from build123d import *

# Parameters (mm, degrees)
SKETCH1_R           = 1.75
BOSS_EXTRUDE1_DEPTH = 3
SKETCH2_W           = 5
SKETCH2_H           = 8
BOSS_EXTRUDE2_DEPTH = 12
BOSS_EXTRUDE3_DEPTH = 8
FILLET2_R           = 8


with BuildPart() as part:
    # Sketch1 → Boss-Extrude1 (new body)
    with BuildSketch(Plane(origin=(0, 0, 0), x_dir=(1, 0, 0), z_dir=(0, 1, 0))):
        with BuildLine():
            Line((-11.25, -4), (11.25, -4))
            ThreePointArc((11.25, -4), (15.25, 0), (11.25, 4))
            Line((11.25, 4), (-11.25, 4))
            ThreePointArc((-11.25, 4), (-15.25, 0), (-11.25, -4))
        make_face()
        with Locations((-11.25, 0)):
            Circle(SKETCH1_R, mode=Mode.SUBTRACT)
        with Locations((11.25, 0)):
            Circle(SKETCH1_R, mode=Mode.SUBTRACT)
    extrude(amount=BOSS_EXTRUDE1_DEPTH)

    # Sketch2 → Boss-Extrude2 (add)
    with BuildSketch(Plane(origin=(0, 3, 0), x_dir=(1, 0, 0), z_dir=(0, 1, 0))):
        with Locations((3.75, 0)):
            Rectangle(SKETCH2_W, SKETCH2_H)
    extrude(amount=BOSS_EXTRUDE2_DEPTH)

    # Sketch3 → Boss-Extrude3 (add)
    with BuildSketch(Plane.XY.offset(4)):
        Polygon((1.25, 15), (-6.25, 3), (1.25, 3), align=None)
    extrude(amount=-BOSS_EXTRUDE3_DEPTH)

    # Fillet2
    fillet2_edges = [part.edges().sort_by_distance(p)[0] for p in [
        (1.25, 15, 0),
    ]]
    fillet(fillet2_edges, radius=FILLET2_R)


solid = part.part
For this review, take the finished solid that the model builds, in its own axes (mm). A direction names the side the tool comes from. Give positions to 0.01 mm unless a question says otherwise; leave off trailing zeros. Loops run counter-clockwise (first coordinate to the right, second up) from the corner with the lowest first, then second, coordinate; pieces in that order, holes last. Notation, with made-up numbers: M 52.5,10.25 L 59.5,10.25 A20 cw 59.5,22.25 Z; hole C 21,47 d9. An arc over 180 degrees is marked long. Answer as a JSON object with one key per item and string values. Group by question number.
Q1. Add section C-C on z = 0. Give the boundary of the cut face in (x, y), and give its area (3 significant figures).
Q2. Add section B-B on x = -10.5. Give the boundary of the cut face in (y, z).
Q3. Mouldability with a two-part tool opening along X and no side actions: class faces 4 (the cylindrical face through (12.919, 1.479, -0.526)), 5 (the flat face through (-3.639, 7.178, 0.056)), 6 (the flat face through (6.25, 9, 0)), 7 (the flat face through (0, 6, 4)) as +X half, -X half, draft (parallel to the pull), parting line (faces both ways), or undercut.
Q4. For probe 1 along X at (y, z) = (2.1, 0); probe 2 along Z at (x, y) = (-11.25, 1.05); probe 3 along Y at (x, z) = (12.5, -3.5), list the stretches that pass through material, from the lowest coordinate up. Write a range as [from, to].
Q5. Insertion check: P1, Ø2, axis at x = 10, z = -2, coming from the -Y side; P2, Ø3, axis at x = -2, z = -1.5, coming from the +Y side; P3, Ø4, axis at x = 11.25, z = 0, coming from the +Y side; P4, Ø1, axis at y = 4, z = -1.5, coming from the -X side. Each pin has a flat end and moves straight along its axis. Give the tip position at first contact, or say it passes through.
Q6. Tool access review of faces 1 (the flat face through (-9, 3, 0)), 2 (the flat face through (9, 3, 0)), 3 (the flat face through (0, 0, 0)): name each direction out of +Z, -Z, +X, -X, +Y, -Y from which nothing blocks a thin tool from reaching the whole face with its end or side.
Q7. Add section D-D on x = -4.5. Give the boundary of the cut face in (y, z), and give its area (3 significant figures).
Q8. Add section A-A on y = 2.25. Give the boundary of the cut face in (x, z), and give its area (3 significant figures).
Checked values:
{
 "1": {"outline": "M -15.25,0 L -13,0 L -13,3 L -15.25,3 Z; M -9.5,0 L 9.5,0 L 9.5,3 L 6.25,3 L 6.25,15 L 5.68,15 A8 ccw -1.1,11.24 L -6.25,3 L -9.5,3 Z; M 13,0 L 15.25,0 L 15.25,3 L 13,3 Z", "area": "172 mm²"},
 "2": {"outline": "M 0,-4 L 3,-4 L 3,-1.58 L 0,-1.58 Z; M 0,1.58 L 3,1.58 L 3,4 L 0,4 Z"},
 "3": {"face 4": "undercut", "face 5": "-X half", "face 6": "+X half", "face 7": "draft"},
 "4": {"probe 1": "[-15.25, -13], [-9.5, 9.5], [13, 15.25]", "probe 2": "[-4, -1.75], [1.75, 4]", "probe 3": "[0, 3]"},
 "5": {"P1": "y = 0", "P2": "y = 12.08", "P3": "y = 3", "P4": "x = -5.94"},
 "6": {"face 1": "+Z, -Z, -X, +Y", "face 2": "+Z, -Z, +X, +Y", "face 3": "+Z, -Z, +X, -X, -Y"},
 "7": {"outline": "M 0,-4 L 5.8,-4 L 5.8,4 L 0,4 Z", "area": "46.4 mm²"},
 "8": {"outline": "M -11.25,-4 L 11.25,-4 A4 ccw 11.25,4 L -11.25,4 A4 ccw Z; hole C -11.25,0 d3.5; hole C 11.25,0 d3.5", "area": "211 mm²"}
}
